from build123d import *

# Parameters (mm, degrees)
SKETCH1_W           = 110
SKETCH1_H           = 58
BOSS_EXTRUDE1_DEPTH = 2.5
SKETCH2_W           = 104.8
SKETCH2_H           = 52.8
BOSS_EXTRUDE2_DEPTH = 1.5
SKETCH3_W           = 5
SKETCH3_H           = 2
BOSS_EXTRUDE3_DEPTH = 3
FILLET1_R           = 1
SKETCH4_W           = 6
SKETCH4_H           = 2.6
CUT_EXTRUDE1_DEPTH  = 1
FILLET2_R           = 1
CHAMFER1_SIZE       = 0.5
CUT_EXTRUDE2_DEPTH  = 125.551194294
FILLET3_R           = 1


with BuildPart() as part:
    # Sketch1 → Boss-Extrude1 (new body)
    with BuildSketch(Plane(origin=(0, 0, 0), x_dir=(1, 0, 0), z_dir=(0, 1, 0))):
        with Locations((55, 29)):
            Rectangle(SKETCH1_W, SKETCH1_H)
    extrude(amount=BOSS_EXTRUDE1_DEPTH)

    # Sketch2 → Boss-Extrude2 (add)
    with BuildSketch(Plane.XZ):
        with Locations((55, -29)):
            Rectangle(SKETCH2_W, SKETCH2_H)
    extrude(amount=BOSS_EXTRUDE2_DEPTH)

    # Sketch3 → Boss-Extrude3 (add)
    with BuildSketch(Plane.XZ.offset(1.5)):
        with Locations((55, -3.6)):
            Rectangle(SKETCH3_W, SKETCH3_H)
        Polygon((2.6, -2.6), (7.6, -2.6), (7.6, -4.6), (4.6, -4.6), (4.6, -7.6), (2.6, -7.6), align=None)
        Polygon((107.4, -2.6), (107.4, -7.6), (105.4, -7.6), (105.4, -4.6), (102.4, -4.6), (102.4, -2.6), align=None)
        Polygon((107.4, -55.4), (102.4, -55.4), (102.4, -53.4), (105.4, -53.4), (105.4, -50.4), (107.4, -50.4), align=None)
        with Locations((55, -54.4)):
            Rectangle(SKETCH3_W, SKETCH3_H)
        Polygon((2.6, -55.4), (2.6, -50.4), (4.6, -50.4), (4.6, -53.4), (7.6, -53.4), (7.6, -55.4), align=None)
    extrude(amount=BOSS_EXTRUDE3_DEPTH)

    # Fillet1
    fillet1_edges = [part.edges().sort_by_distance(p)[0] for p in [
        (105.4, -3, -53.4),
        (4.6, -3, -4.6),
        (105.4, -3, -4.6),
        (4.6, -3, -53.4),
    ]]
    fillet(fillet1_edges, radius=FILLET1_R)

    # Sketch4 → Cut-Extrude1 (cut)
    with BuildSketch(Plane.XZ):
        with Locations((27.5, -1.3)):
            Rectangle(SKETCH4_W, SKETCH4_H)
        with Locations((82.5, -1.3)):
            Rectangle(SKETCH4_W, SKETCH4_H)
        with Locations((82.5, -56.7)):
            Rectangle(SKETCH4_W, SKETCH4_H)
        with Locations((27.5, -56.7)):
            Rectangle(SKETCH4_W, SKETCH4_H)
    extrude(amount=-CUT_EXTRUDE1_DEPTH, mode=Mode.SUBTRACT)

    # Fillet2
    fillet2_edges = [part.edges().sort_by_distance(p)[0] for p in [
        (0, 1.25, -58),
        (110, 1.25, -58),
        (110, 1.25, 0),
        (0, 1.25, 0),
    ]]
    fillet(fillet2_edges, radius=FILLET2_R)

    # Chamfer1
    chamfer1_edges = [part.edges().sort_by_distance(p)[0] for p in [
        (55, -4.5, -55.4),
        (2.6, -3, -50.4),
        (2.6, -2.25, -55.4),
        (7.6, -3, -55.4),
        (107.4, -3, -50.4),
        (102.4, -3, -55.4),
        (107.4, -2.25, -55.4),
        (107.4, -2.25, -2.6),
        (107.4, -4.5, -5.1),
        (104.9, -4.5, -2.6),
        (55, -4.5, -2.6),
        (2.6, -4.5, -5.1),
        (5.1, -4.5, -2.6),
        (2.6, -2.25, -2.6),
    ]]
    chamfer(chamfer1_edges, length=CHAMFER1_SIZE)

    # Sketch5 → Cut-Extrude2 (cut, through all)
    with BuildSketch(Plane(origin=(0, 2.5, 0), x_dir=(1, 0, 0), z_dir=(0, 1, 0))):
        with BuildLine():
            Line((56.5, 46.5), (56.5, 11.5))
            ThreePointArc((56.5, 11.5), (55, 10), (53.5, 11.5))
            Line((53.5, 11.5), (53.5, 46.5))
            ThreePointArc((53.5, 46.5), (55, 48), (56.5, 46.5))
        make_face()
        with BuildLine():
            Line((67.5, 46.5), (67.5, 11.5))
            ThreePointArc((67.5, 11.5), (69, 10), (70.5, 11.5))
            Line((70.5, 11.5), (70.5, 46.5))
            ThreePointArc((70.5, 46.5), (69, 48), (67.5, 46.5))
        make_face()
        with BuildLine():
            Line((81.5, 46.5), (81.5, 11.5))
            ThreePointArc((81.5, 11.5), (83, 10), (84.5, 11.5))
            Line((84.5, 11.5), (84.5, 46.5))
            ThreePointArc((84.5, 46.5), (83, 48), (81.5, 46.5))
        make_face()
        with BuildLine():
            Line((95.5, 46.5), (95.5, 11.5))
            ThreePointArc((95.5, 11.5), (97, 10), (98.5, 11.5))
            Line((98.5, 11.5), (98.5, 46.5))
            ThreePointArc((98.5, 46.5), (97, 48), (95.5, 46.5))
        make_face()
        with BuildLine():
            Line((39.5, 46.5), (39.5, 11.5))
            ThreePointArc((39.5, 11.5), (41, 10), (42.5, 11.5))
            Line((42.5, 11.5), (42.5, 46.5))
            ThreePointArc((42.5, 46.5), (41, 48), (39.5, 46.5))
        make_face()
        with BuildLine():
            Line((25.5, 46.5), (25.5, 11.5))
            ThreePointArc((25.5, 11.5), (27, 10), (28.5, 11.5))
            Line((28.5, 11.5), (28.5, 46.5))
            ThreePointArc((28.5, 46.5), (27, 48), (25.5, 46.5))
        make_face()
        with BuildLine():
            Line((11.5, 46.5), (11.5, 11.5))
            ThreePointArc((11.5, 11.5), (13, 10), (14.5, 11.5))
            Line((14.5, 11.5), (14.5, 46.5))
            ThreePointArc((14.5, 46.5), (13, 48), (11.5, 46.5))
        make_face()
    extrude(amount=-CUT_EXTRUDE2_DEPTH, mode=Mode.SUBTRACT)

    # Fillet3
    fillet3_edges = [part.edges().sort_by_distance(p)[0] for p in [
        (0, 2.5, -29),
        (55, 2.5, -58),
        (55, 2.5, 0),
        (110, 2.5, -29),
        (109.707106781, 2.5, -0.292893219),
        (109.707106781, 2.5, -57.707106781),
        (0.292893219, 2.5, -0.292893219),
        (0.292893219, 2.5, -57.707106781),
    ]]
    fillet(fillet3_edges, radius=FILLET3_R)


solid = part.part
Verification items for the finished model (mm, model axes). A direction names the side the tool comes from. Coordinates: 2 decimals unless noted, no trailing zeros. Order: outer loops, then holes, each group sorted by start corner. A loop starts at its lowest first (then second) coordinate and runs counter-clockwise, first axis right, second up. Notation, with made-up numbers: (11, 5) -> (55, 5) arc R20 cw to (55, 34) -> close; hole circle Ø2 at (-17, 53). An arc over 180 degrees is marked (long way). Put each result on its own line as item: value. Start each with the question number.
1. Cross-section at A-A, the plane x = 97. Record the boundary of the cut face in (y, z), then the cut area to 3 significant figures.
2. Go/stop test with flat-tipped pins: pin 1 Ø0.6 at (y, z) = (-2.5, -51) entering from -X; pin 2 Ø1 at (x, z) = (72, -21.5) entering from -Y; pin 3 Ø1 at (x, y) = (7, -3) entering from -Z. Record where each tip stops, or that it passes through.
3. Cross-section at B-B, the plane x = 27. Record the boundary of the cut face in (y, z).
4. Mould release check, pull along Z, two halves, no side actions. Record for faces 4 (the flat face through (70.5, 1, -29)), 5 (the flat face through (66, 2.5, -29)): released by +Z, released by -Z, zero draft, split by the parting line, or undercut.
5. Material ranges on L1, parallel to X at y = -1.75, z = -54; L2, parallel to X at y = -1.25, z = -5; L3, parallel to Y at x = 89, z = -46, recorded low to high. Write a range as [from, to].
6. Cross-section at C-C, the plane z = -35. Count the separate pieces of the cut face and the enclosed holes in it, then the cut area to 3 significant figures.
7. Access from +Z, -Z, +X, -X, +Y, -Y to the whole of each face (thin tool, end or side, straight path). Record for faces 1 (the cylindrical face through (27, 1, -10)), 2 (the flat face through (55, 0, -57)), 3 (the flat face through (108, 0, -29)).
Computed:
1. outline: (-1.5, -55.4) -> (0, -55.4) -> (0, -58) -> (1.5, -58) arc R1 ccw to (2.5, -57) -> (2.5, -48) -> (-1.5, -48) -> close; (-1.5, -10) -> (2.5, -10) -> (2.5, -1) arc R1 ccw to (1.5, 0) -> (0, 0) -> (0, -2.6) -> (-1.5, -2.6) -> close
1. area: 71.8 mm2
2. pin 1: x = 2.6
2. pin 2: y = -1.5
2. pin 3: z = -55.4
3. outline: (-1.5, -55.4) -> (1, -55.4) -> (1, -58) -> (1.5, -58) arc R1 ccw to (2.5, -57) -> (2.5, -48) -> (-1.5, -48) -> close; (-1.5, -10) -> (2.5, -10) -> (2.5, -1) arc R1 ccw to (1.5, 0) -> (1, 0) -> (1, -2.6) -> (-1.5, -2.6) -> close
4. face 4: undercut
4. face 5: zero draft
5. L1: [2.6, 7.6], [52.5, 57.5], [102.4, 107.4]
5. L2: [2.6, 107.4]
5. L3: [-1.5, 2.5]
6. separate pieces: 8
6. enclosed holes: 0
6. area: 348 mm2
7. face 1: +Y, -Y
7. face 2: -Z, +X, -X, -Y
7. face 3: +X, -Y
